Geometry check sheet. Reference: the model listing, model coordinates, mm. A direction names the side the tool comes from. Coordinates: 2 decimals unless noted, no trailing zeros. Write each loop counter-clockwise with the first axis right and the second up, starting at its lowest first coordinate (ties: lowest second). Pieces come first, ordered by that corner, then holes. Notation, with made-up numbers: (-38.75, -17.5) - (5.25, -17.5) arc R22 ccw to (5.25, -9.5) - close; hole circle Ø1 at (23, 4). An arc over 180 degrees is marked (long way). Answer as a JSON object with one key per item and string values. Group by question number.
from build123d import *

# Parameters (mm, degrees)
SKETCH1_R           = 12.7
BOSS_EXTRUDE1_DEPTH = 30.1625
SKETCH4_R           = 25.4
BOSS_EXTRUDE2_DEPTH = 50.00625
CUT_EXTRUDE1_DEPTH  = 11.176
SKETCH3_R           = 6
CUT_EXTRUDE2_DEPTH  = 8
SKETCH5_R           = 3.175
BOSS_EXTRUDE3_DEPTH = 6.604
CUT_EXTRUDE3_START  = -6.35
SKETCH9_R           = 25.4
SKETCH9_R_2         = 6.35
CUT_EXTRUDE3_DEPTH  = 38.1
CUT_EXTRUDE4_REACH  = 58.61
SKETCH10_R          = 25.4
SKETCH10_R_2        = 22.225
FILLET1_R           = 3.175
CHAMFER1_SIZE       = 1.27


with BuildPart() as part:
    # Sketch1 → Boss-Extrude1 (new body)
    with BuildSketch(Plane(origin=(0, 0, 0), x_dir=(1, 0, 0), z_dir=(0, 1, 0))):
        Circle(SKETCH1_R)
    extrude(amount=BOSS_EXTRUDE1_DEPTH)

    # Sketch4 → Boss-Extrude2 (add)
    with BuildSketch(Plane(origin=(0, 30.1625, 0), x_dir=(1, 0, 0), z_dir=(0, 1, 0))):
        Circle(SKETCH4_R)
    extrude(amount=BOSS_EXTRUDE2_DEPTH)

    # Sketch2 → Cut-Extrude1 (cut)
    with BuildSketch(Plane.XZ):
        with BuildLine():
            Line((-7, 2.899494937), (-8.776962921, 1.122532015))
            ThreePointArc((-8.776962921, 1.122532015), (-9.241930906, 0), (-8.776962921, -1.122532015))
            Line((-8.776962921, -1.122532015), (-7, -2.899494937))
            Line((-7, -2.899494937), (-7, 2.899494937))
        make_face()
        Polygon((-2.899494937, 7), (-7, 2.899494937), (-7, -2.899494937), (-2.899494937, -7), (2.899494937, -7), (7, -2.899494937), (7, 2.899494937), (2.899494937, 7), align=None)
        with BuildLine():
            Line((-7, 5.4125), (-7, 2.899494937))
            Line((-7, 2.899494937), (-2.899494937, 7))
            Line((-2.899494937, 7), (-5.4125, 7))
            ThreePointArc((-5.4125, 7), (-6.535032015, 6.535032015), (-7, 5.4125))
        make_face()
        with BuildLine():
            Line((-1.122532015, 8.776962921), (-2.899494937, 7))
            Line((-2.899494937, 7), (2.899494937, 7))
            Line((2.899494937, 7), (1.122532015, 8.776962921))
            ThreePointArc((1.122532015, 8.776962921), (0, 9.241930906), (-1.122532015, 8.776962921))
        make_face()
        with BuildLine():
            Line((5.4125, 7), (2.899494937, 7))
            Line((2.899494937, 7), (7, 2.899494937))
            Line((7, 2.899494937), (7, 5.4125))
            ThreePointArc((7, 5.4125), (6.535032015, 6.535032015), (5.4125, 7))
        make_face()
        with BuildLine():
            Line((8.776962921, 1.122532015), (7, 2.899494937))
            Line((7, 2.899494937), (7, -2.899494937))
            Line((7, -2.899494937), (8.776962921, -1.122532015))
            ThreePointArc((8.776962921, -1.122532015), (9.241930906, 0), (8.776962921, 1.122532015))
        make_face()
        with BuildLine():
            Line((7, -2.899494937), (2.899494937, -7))
            Line((2.899494937, -7), (5.4125, -7))
            ThreePointArc((5.4125, -7), (6.535032015, -6.535032015), (7, -5.4125))
            Line((7, -5.4125), (7, -2.899494937))
        make_face()
        with BuildLine():
            Line((2.899494937, -7), (-2.899494937, -7))
            Line((-2.899494937, -7), (-1.122532015, -8.776962921))
            ThreePointArc((-1.122532015, -8.776962921), (0, -9.241930906), (1.122532015, -8.776962921))
            Line((1.122532015, -8.776962921), (2.899494937, -7))
        make_face()
        with BuildLine():
            Line((-2.899494937, -7), (-7, -2.899494937))
            Line((-7, -2.899494937), (-7, -5.4125))
            ThreePointArc((-7, -5.4125), (-6.535032015, -6.535032015), (-5.4125, -7))
            Line((-5.4125, -7), (-2.899494937, -7))
        make_face()
    extrude(amount=-CUT_EXTRUDE1_DEPTH, mode=Mode.SUBTRACT)

    # Sketch3 → Cut-Extrude2 (cut)
    with BuildSketch(Plane.XZ.offset(-11.176)):
        Circle(SKETCH3_R)
    extrude(amount=-CUT_EXTRUDE2_DEPTH, mode=Mode.SUBTRACT)

    # Sketch5 → Boss-Extrude3 (add)
    with BuildSketch(Plane(origin=(0, 80.16875, 0), x_dir=(1, 0, 0), z_dir=(0, 1, 0))):
        Circle(SKETCH5_R)
    extrude(amount=BOSS_EXTRUDE3_DEPTH)

    # Sketch9 → Cut-Extrude3 (cut)
    with BuildSketch(Plane(origin=(0, 80.16875, 0), x_dir=(1, 0, 0), z_dir=(0, 1, 0)).offset(CUT_EXTRUDE3_START)):
        Circle(SKETCH9_R)
        Circle(SKETCH9_R_2, mode=Mode.SUBTRACT)
    extrude(amount=-CUT_EXTRUDE3_DEPTH, mode=Mode.SUBTRACT)

    # Sketch10 → Cut-Extrude4 (cut, up to next)
    with BuildSketch(Plane.XZ.offset(-30.1625), mode=Mode.PRIVATE) as cut_extrude4_sk1:
        Circle(SKETCH10_R)
        Circle(SKETCH10_R_2, mode=Mode.SUBTRACT)
    cut_extrude4_tool1 = extrude(cut_extrude4_sk1.sketch, amount=-CUT_EXTRUDE4_REACH, mode=Mode.PRIVATE) & part.part
    add(cut_extrude4_tool1.solids().sort_by_distance((-24.68158, 30.1625, 0))[0], mode=Mode.SUBTRACT)

    # Fillet1
    fillet1_edges = [part.edges().sort_by_distance(p)[0] for p in [
        (-6.35, 35.71875, 0),
        (-6.35, 73.81875, 0),
    ]]
    fillet(fillet1_edges, radius=FILLET1_R)

    # Chamfer1
    chamfer1_edges = [part.edges().sort_by_distance(p)[0] for p in [
        (-25.4, 73.81875, 0),
        (-22.225, 30.1625, 0),
    ]]
    chamfer(chamfer1_edges, length=CHAMFER1_SIZE)


solid = part.part
(1) Draft check along X on faces 1 (the face through (-0.69, 83.42, 3.1)), 2 (the face through (0, 35.719, 10)), 3 (the face through (-7.9, 5.5, -2)). Enter one of: +X half, -X half, draft (parallel to the pull), parting line (faces both ways), or undercut.
(2) Section check C-C (y = 33). Record the cut outline in (x, z) (3 decimals), and give its area (3 significant figures).
(3) Section check B-B (y = 49). Record the cut outline in (x, z).
(4) Section check A-A (y = 15). Record the cut outline in (x, z).
(5) Material ranges on L1, parallel to Z at x = 0, y = 17.25; L2, parallel to Y at x = 10, z = 0; L3, parallel to Y at x = -14.5, z = 14, recorded low to high. Write a range as [from, to].
(6) Gauge pin test, flat ends, axial feed: pin 1 (3 mm diameter, centred on y = 7, z = -3.5, fed in from -X); pin 2 (15 mm diameter, centred on x = -2, z = -2, fed in from -Y); pin 3 (2 mm diameter, centred on x = 4, y = 8, fed in from -Z); pin 4 (10 mm diameter, centred on x = -2, z = -10.5, fed in from +Y). Record the tip position at first contact, or that the pin passes through.
(7) Set-up check for faces 4 (the face through (4, 6, 7)), 5 (the face through (0, 73.819, 10)): record each of +Z, -Z, +X, -X, +Y, -Y from which the full face is reachable in a straight line by a thin tool's end or side.
Conclusion:
{
 "1": {"face 1": "parting line", "face 2": "draft", "face 3": "undercut"},
 "2": {"outline": "circle Ø44.45 at (0, 0)", "area": "1,550 mm^2"},
 "3": {"outline": "circle Ø12.7 at (0, 0)"},
 "4": {"outline": "circle Ø25.4 at (0, 0); hole circle Ø12 at (0, 0)"},
 "5": {"L1": "z = [-12.7, -6], [6, 12.7]", "L2": "y = [0, 35.72], [73.82, 80.17]", "L3": "y = [30.16, 35.72], [73.82, 80.17]"},
 "6": {"pin 1": "stops at x = -12.54", "pin 2": "stops at y = 0", "pin 3": "stops at z = -12.34", "pin 4": "stops at y = 80.17"},
 "7": {"face 4": "-Y", "face 5": "none"}
}
